Here's how the part is built. I have some questions about the finished solid (model axes, mm). Coordinates: 2 decimals unless noted, no trailing zeros. Write each loop counter-clockwise with the first axis right and the second up, starting at its lowest first coordinate (ties: lowest second). Pieces come first, ordered by that corner, then holes. Notation, with made-up numbers: (-10, 22) -> (4, 22) arc R17 ccw to (4, 38) -> close; hole circle Ø9 at (-10, -9.5). An arc over 180 degrees is marked (long way). Answer in a Markdown table with one row per item. Add a question column.
Autodesk Inventor part; units mm, degrees
ref_plane "YZ Plane" through (0, 0, 0) normal (1, 0, 0) x (0, 1, 0)
ref_plane "XZ Plane" through (0, 0, 0) normal (0, 1, 0) x (-1, 0, 0)
ref_plane "XY Plane" through (0, 0, 0) normal (0, 0, 1) x (1, 0, 0)
sketch "Sketch1" plane through (0, 0, 0) normal (0, 0, 1) x (1, 0, 0)
  line L0 (-7.3323, 0) -> (-3.6662, 6.35)
  line L1 (-3.6662, 6.35) -> (3.6662, 6.35)
  line L2 (3.6662, 6.35) -> (7.3323, 0)
  line L3 (7.3323, 0) -> (3.6662, -6.35)
  line L4 (3.6662, -6.35) -> (-3.6662, -6.35)
  line L5 (-3.6662, -6.35) -> (-7.3323, 0)
  point P0 (0, 0)
  point P1 (0, 0)
  dimension "d0" = 12.7
extrude "Extrusion1" add sketch "Sketch1" along normal blind 6.35
sketch "Sketch2" plane through (0, 0, 6.35) normal (0, 0, 1) x (1, 0, 0)
  circle A0 centre (0, 0) radius 3.175
  dimension "d3" = 6.35
extrude "Extrusion2" cut sketch "Sketch2" against normal blind 6.35
thread "Thread1"
fillet "Fillet1" radius 3.175 6 edges at (0, 6.35, 6.35) (5.4993, 3.175, 6.35) (-5.4993, 3.175, 6.35) (-5.4993, -3.175, 6.35) (0, -6.35, 6.35) (5.4993, -3.175, 6.35)
properties part number "LucasCharles Part 8 small nut Final" material "Stainless Steel, Austenitic"
Q1. I'm going to push flat-ended pins straight in: P1, Ø3, axis at x = -3, y = -2.5, coming from the -Z side; P2, Ø2, axis at x = -5, y = -1, coming from the +Z side. Where does each tip first touch, or does it pass through?
Q2. I need wall thicknesses on line 1 (Y direction, x = 0, z = 3.25) (3 decimals); line 2 (Y direction, x = 0, z = 2) (3 decimals); line 3 (X direction, y = 0.5, z = 2.75). Which ranges of each line are inside material? Lowest first, please. Write a range as [from, to].
Q3. Imagine slicing it at C-C on z = 5.25. Please give me the cut outline in (x, y) (3 decimals), plus the area to 3 significant figures.
Q4. If we mould it in two halves opening along Y, with no side actions, what happens to faces 1 (the cylindrical face through (0.051, 5.796, 4.968)), 2 (the cylindrical face through (4.994, -2.942, 4.968)), 3 (the cylindrical face through (-0.69, -3.1, 3.22))? For each: pulls with the +Y half, pulls with the -Y half, needs draft (parallel to the pull), parting line crosses it, or undercut.
Q5. Imagine slicing it at B-B on z = 2. Please give me the cut outline in (x, y) (3 decimals), plus the area to 3 significant figures.
Result sheet:
| question | item | result |
|---|---|---|
| 1 | P1 | stops at z = 0 |
| 1 | P2 | stops at z = 6.28 |
| 2 | line 1 | y = [-6.349, -3.175], [3.175, 6.349] |
| 2 | line 2 | y = [-6.35, -3.175], [3.175, 6.35] |
| 2 | line 3 | x = [-7.04, -3.14], [3.14, 7.04] |
| 3 | outline | (-6.441, 0) -> (-3.221, -5.578) -> (3.221, -5.578) -> (6.441, 0) -> (3.221, 5.578) -> (-3.221, 5.578) -> close; hole circle Ø6.35 at (0, 0) |
| 3 | area | 76.1 mm^2 |
| 4 | face 1 | pulls with the +Y half |
| 4 | face 2 | pulls with the -Y half |
| 4 | face 3 | undercut |
| 5 | outline | (-7.332, 0) -> (-3.666, -6.35) -> (3.666, -6.35) -> (7.332, 0) -> (3.666, 6.35) -> (-3.666, 6.35) -> close; hole circle Ø6.35 at (0, 0) |
| 5 | area | 108 mm^2 |
